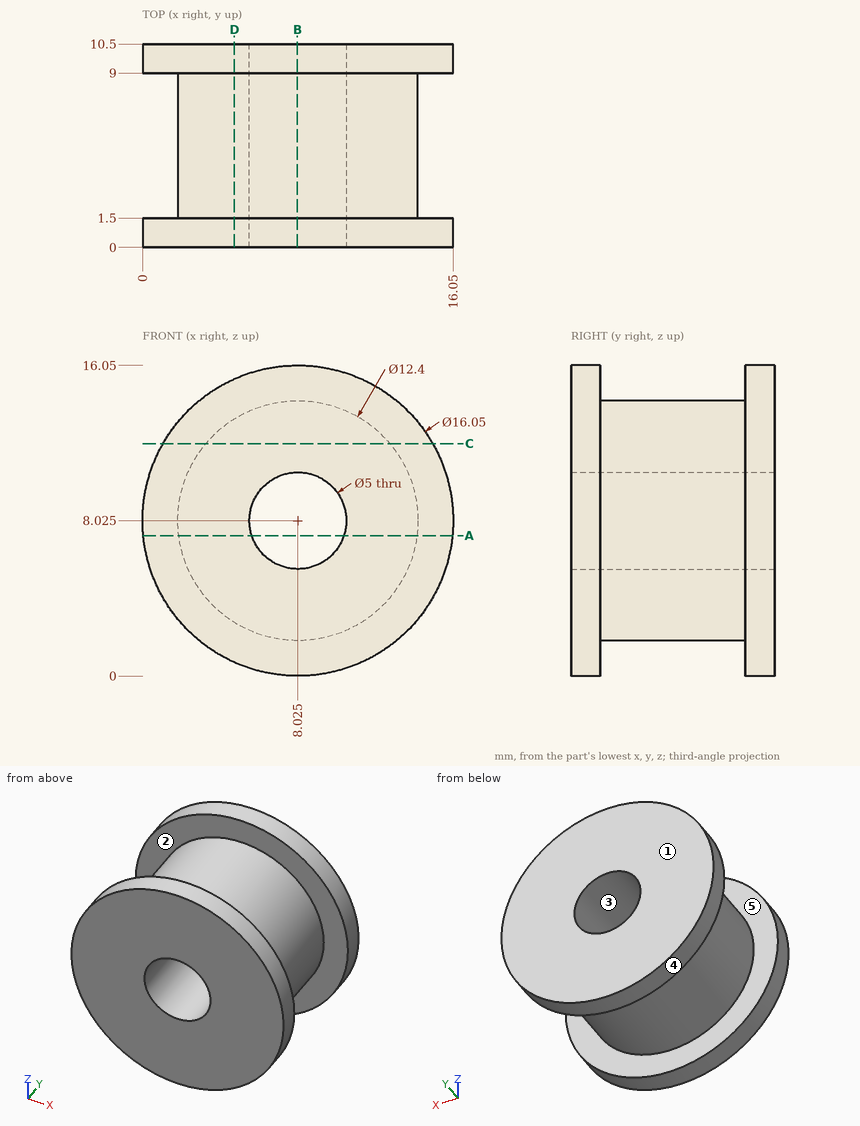
Can you work these out from the drawing? Everything is in mm from the part's minimum corner. A direction names the side the tool comes from. Round coordinates to 2 decimals unless told otherwise and drop trailing zeros. Loops run counter-clockwise (first coordinate to the right, second up) from the corner with the lowest first, then second, coordinate; pieces in that order, holes last. Notation, with made-up numbers: M 81.5,29 L 86.5,29 A25 cw 86.5,64 Z; hole C -13,0 d3. An arc over 180 degrees is marked long. Write item = value, one per line.
1. I want a section at C-C, the plane z = 12. Write out the boundary of the cut face in (x, y), and give its area (3 significant figures).
Results below:
outline = M 1.05,0 L 15,0 L 15,1.5 L 12.78,1.5 L 12.78,9 L 15,9 L 15,10.5 L 1.05,10.5 L 1.05,9 L 3.27,9 L 3.27,1.5 L 1.05,1.5 Z
area = 113 mm²
2. Which directions (+Z, -Z, +X, -X, +Y, -Y) give clear straight access to the entire face, cutting with the end or side of a thin tool? Please do the marked faces 1 and 2.
Results below:
face_1 = +Z, -Z, +X, -X, +Y
face_2 = none
3. I need wall thicknesses on probe 1 along Y at (x, z) = (3.75, 3.25); probe 2 along Z at (x, y) = (8, 6.75); probe 3 along Z at (x, y) = (10.25, 4.5). Which ranges of each line are inside material? Lowest first, please.
Results below:
probe_1 = 0 to 1.5, 9 to 10.5
probe_2 = 1.83 to 5.53, 10.52 to 14.22
probe_3 = 2.24 to 6.89, 9.16 to 13.81
4. Thinking about a two-plate mould opening in X: for the marked faces 3, 4 and 5, which applies, +X half, -X half, draft (parallel to the pull), parting line (faces both ways), or undercut?
Results below:
face_3 = undercut
face_4 = parting line
face_5 = draft
5. Will these pins go through, and if not, where does the flat tip stop? P1, Ø6, axis at x = 12, y = 7.5, coming from the -Z side; P2, Ø5, axis at y = 2, z = 12.5, coming from the +X side.
Results below:
P1 = 0.12
P2 = 15.79
6. I want a section at D-D, the plane x = 4.75. Write out the boundary of the cut face in (y, z).
Results below:
outline = M 0,0.7 L 1.5,0.7 L 1.5,2.76 L 9,2.76 L 9,0.7 L 10.5,0.7 L 10.5,15.35 L 9,15.35 L 9,13.29 L 1.5,13.29 L 1.5,15.35 L 0,15.35 Z
7. I want a section at A-A, the plane z = 7.25. Write out the boundary of the cut face in (x, y), and give its area (3 significant figures).
Results below:
outline = M 0.04,0 L 5.65,0 L 5.65,10.5 L 0.04,10.5 L 0.04,9 L 1.87,9 L 1.87,1.5 L 0.04,1.5 Z; M 10.4,0 L 16.01,0 L 16.01,1.5 L 14.18,1.5 L 14.18,9 L 16.01,9 L 16.01,10.5 L 10.4,10.5 Z
area = 90.3 mm²
8. I want a section at B-B, the plane x = 8. Write out the boundary of the cut face in (y, z), and give its area (3 significant figures).
Results below:
outline = M 0,0 L 1.5,0 L 1.5,1.83 L 9,1.83 L 9,0 L 10.5,0 L 10.5,5.53 L 0,5.53 Z; M 0,10.52 L 10.5,10.52 L 10.5,16.05 L 9,16.05 L 9,14.22 L 1.5,14.22 L 1.5,16.05 L 0,16.05 Z
area = 88.7 mm²
